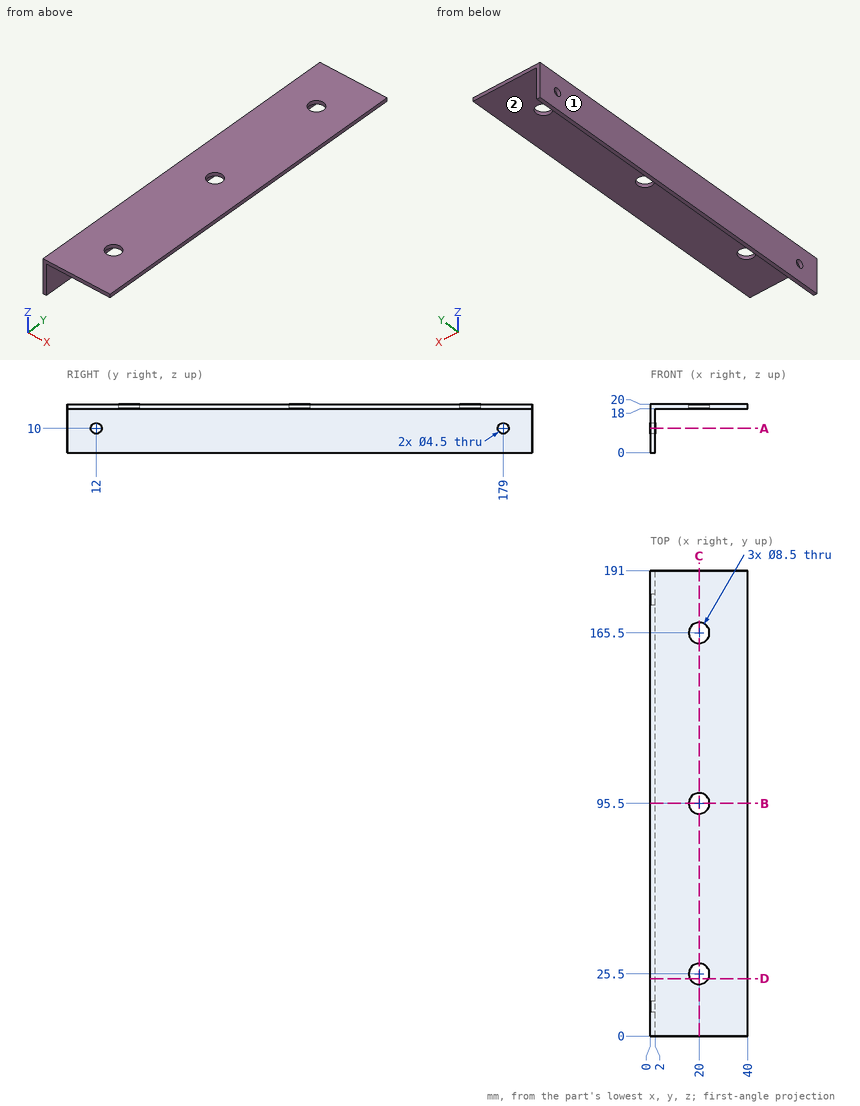
Input: dimensioned drawing with shaded views. Units: mm. Origin: part minimum x, y, z. A direction names the side the tool comes from. Round coordinates to 2 decimals unless told otherwise and drop trailing zeros. Write each loop counter-clockwise with the first axis right and the second up, starting at its lowest first coordinate (ties: lowest second). Pieces come first, ordered by that corner, then holes. Notation, with made-up numbers: (30.25, 64.25) - (70.25, 64.25) arc R28 ccw to (70.25, 102.25) - close; hole circle Ø4 at (-18.5, -7.5). An arc over 180 degrees is marked (long way). Write item = value, one per line.
(1) Section query B-B on y = 95.5. Output: boundary loops of the cut face in (x, z), then the cut area to 3 significant figures.
Geometry check:
outline = (0, 0) - (2, 0) - (2, 18) - (15.75, 18) - (15.75, 20) - (0, 20) - close; (24.25, 18) - (40, 18) - (40, 20) - (24.25, 20) - close
area = 99.0 mm^2
(2) Section query A-A on z = 10. Output: boundary loops of the cut face in (x, y).
Geometry check:
outline = (0, 0) - (2, 0) - (2, 9.75) - (0, 9.75) - close; (0, 14.25) - (2, 14.25) - (2, 176.75) - (0, 176.75) - close; (0, 181.25) - (2, 181.25) - (2, 191) - (0, 191) - close
(3) Section query C-C on x = 20. Output: boundary loops of the cut face in (y, z), then the cut area to 3 significant figures.
Geometry check:
outline = (0, 18) - (21.25, 18) - (21.25, 20) - (0, 20) - close; (29.75, 18) - (91.25, 18) - (91.25, 20) - (29.75, 20) - close; (99.75, 18) - (161.25, 18) - (161.25, 20) - (99.75, 20) - close; (169.75, 18) - (191, 18) - (191, 20) - (169.75, 20) - close
area = 331 mm^2
(4) Access query for the marked faces 1 and 2. Directions: +Z, -Z, +X, -X, +Y, -Y. A direction counts if a zero-diameter tool reaches every point of the face in a straight line with its end or side. Return the directions, or none.
Geometry check:
face_1 = +Z, -Z, -X, +Y, -Y
face_2 = -Z, +X, +Y, -Y
(5) Contact query for flat-ended pins moving along their axis: pin 1 Ø6 at (y, z) = (38.5, 17) entering from +X; pin 2 Ø3.5 at (y, z) = (179, 10) entering from -X; pin 3 Ø9 at (y, z) = (141.5, 6.5) entering from +X; pin 4 Ø12 at (x, y) = (30.5, 83) entering from -Z. Output: stop coordinate, or through.
Geometry check:
pin_1 = 40
pin_2 = through
pin_3 = 2
pin_4 = 18
(6) Material intervals for probe 1 along Y at (x, z) = (0.7, 10); probe 2 along Y at (x, z) = (20, 18.9); probe 3 along Z at (x, y) = (1.3, 179), sorted ascending.
Geometry check:
probe_1 = 0 to 9.75, 14.25 to 176.75, 181.25 to 191
probe_2 = 0 to 21.25, 29.75 to 91.25, 99.75 to 161.25, 169.75 to 191
probe_3 = 0 to 7.75, 12.25 to 20
(7) Section query D-D on y = 23.5. Output: boundary loops of the cut face in (x, z).
Geometry check:
outline = (0, 0) - (2, 0) - (2, 18) - (16.25, 18) - (16.25, 20) - (0, 20) - close; (23.75, 18) - (40, 18) - (40, 20) - (23.75, 20) - close
